The listing builds one solid part. Answer for the finished solid, in the listing's coordinates (mm). A direction names the side the tool comes from. Coordinates: 2 decimals unless noted, no trailing zeros. Write each loop counter-clockwise with the first axis right and the second up, starting at its lowest first coordinate (ties: lowest second). Pieces come first, ordered by that corner, then holes. Notation, with made-up numbers: M -35,27 L -1,27 A26 ccw -1,42 Z; hole C -30.5,17 d3. An arc over 180 degrees is marked long. Write item = value, one per line. Start each with the question number.
Autodesk Inventor part; units mm, degrees
ref_plane "YZ Plane" through (0, 0, 0) normal (1, 0, 0) x (0, 1, 0)
ref_plane "XZ Plane" through (0, 0, 0) normal (0, 1, 0) x (-1, 0, 0)
ref_plane "XY Plane" through (0, 0, 0) normal (0, 0, 1) x (1, 0, 0)
sketch "Sketch14" plane through (0, 0, 0) normal (0, 1, 0) x (-1, 0, 0)
  line L0 (0, 0) -> (0, -45.5)
  line L1 (0, -45.5) -> (-25, -45.5)
  line L2 (-25, -45.5) -> (-25, -40.4)
  line L3 (-25, -40.4) -> (-37, -40.4)
  line L4 (-33, 0) -> (0, 0)
  line L5 (0, 4) -> (4, 4)
  line L6 (4, 4) -> (4, -45.5)
  line L7 (4, -45.5) -> (4, -49.5)
  line L8 (4, -49.5) -> (-25, -49.5)
  line L9 (-37, -40.4) -> (-37, -44.4)
  line L10 (-33, 0) -> (-37, 0)
  line L11 (-37, 0) -> (-37, 4)
  line L12 (-37, 4) -> (0, 4)
  line L13 (-37, -44.4) -> (-29, -44.4)
  line L14 (-29, -44.4) -> (-25, -49.5)
  dimension "d59" = 45.5
  dimension "d60" = 25
  dimension "d61" = 5.1
  dimension "d62" = 12
  dimension "d64" = 4
  dimension "d65" = 4
  dimension "d66" = 4
  dimension "d67" = 4
  dimension "d68" = 8
extrude "Extrusion10" add sketch "Sketch14" along normal blind 35
sketch "Sketch17" plane through (0, 0, 0) normal (0, -1, 0) x (1, 0, 0)
  line L0 (0, -37.9754) -> (25, -40.4)
  line L1 (0, 0) -> (0, -45.5)
  line L2 (0, -37.9754) -> (0, -45.5)
  line L3 (25, -45.5) -> (0, -45.5)
  line L4 (0, -45.5) -> (25, -45.5)
  line L5 (25, -45.5) -> (25, -40.4)
  line L6 (25, -45.5) -> (25, -40.4)
  line L7 (25, -40.4) -> (0, -37.9754)
extrude "Extrusion12" add sketch "Sketch17" against normal blind 2.5
sketch "Sketch18" plane through (25, 0, -49.5) normal (0, 0, -1) x (-1, 0, 0)
  line L0 (25, 2.5) -> (25, 35)
  line L1 (25, 35) -> (-4.7, 35) construction
  line L2 (-4.7, 35) -> (-4.7, 15) construction
  line L3 (-4.7, 15) -> (25, 15) construction
  line L4 (25, 15) -> (25, 35) construction
  point P0 (25, 0)
  point P1 (-4.7, 25)
  dimension "d77" = 29.7
  dimension "d78" = 20
hole "Hole4" at (29.7, 15, -49.5) at (29.7, 25, -49.5) direction (0, 0, 1) diameter 3.5 depth 9.1 counterbore diameter 6 counterbore depth 7
sketch "Sketch19" plane through (-4, 0, 4) normal (0, 0, 1) x (1, 0, 0)
  circle A0 centre (33.7, 25) radius 1.75
  circle A1 centre (33.7, 15) radius 1.75
  point P0 (4, 0)
hole "Hole5" at (29.7, 25, 4) at (29.7, 15, 4) direction (0, 0, -1) diameter 3.5 depth 4 counterbore diameter 6 counterbore depth 2
properties part number "Swivel Arm Servo Holder"
1. The part is cut by section A-A, the plane y = 25. Write down the section's boundary in (x, z), and give its area (3 significant figures).
2. For faces 5 (the face through (19, 17, 0)), 6 (the face through (32, 15, -42.5)), 7 (the face through (25, 19, -43)), determine the directions among +Z, -Z, +X, -X, +Y, -Y from which every point of the face is accessible in a straight line to the end or side of a thin tool.
3. Straight lines are drawn through the part: L1, parallel to Y at x = 29.7, z = 2.8; L2, parallel to X at y = 25, z = -41; L3, parallel to X at y = 15, z = 1.05. For each, find the intervals that lie inside material, in ascending order. Write a range as [from, to].
4. The part is cut by section D-D, the plane x = 29.7. Count the separate pieces of the cut face and the enclosed holes in it, and give its area (4 significant figures).
5. The part is cut by section B-B, the plane x = 18. Write down the section's boundary in (y, z).
6. The part is cut by section C-C, the plane y = 5. Write down the section's boundary in (x, z), and give its area (3 significant figures).
7. Each of these flat-tipped pins is pushed along its axis until it touches: pin 1 (3 mm diameter, centred on x = 29.7, y = 25, fed in from +Z); pin 2 (6.5 mm diameter, centred on x = 34, y = 21, fed in from -Z); pin 3 (3 mm diameter, centred on x = 30.5, y = 14.5, fed in from -Z); pin 4 (5.5 mm diameter, centred on x = 29.7, y = 15, fed in from +Z). Where does it stop, or does it pass through?
8. For a pull along Y with two mould halves and no side action, classify faces 1 (the face through (32, 25, -42.5)), 2 (the face through (26.726, 24.609, -44.349)), 3 (the face through (31, 17, -40.4)), 4 (the face through (-2, 0, -27)) as pulls with the +Y half, pulls with the -Y half, needs draft (parallel to the pull), parting line crosses it, or undercut.
Solution:
q1.outline = M -4,-49.5 L 25,-49.5 L 26.7,-47.33 L 26.7,-42.5 L 27.95,-42.5 L 27.95,-40.4 L 25,-40.4 L 25,-45.5 L 0,-45.5 L 0,0 L 27.95,0 L 27.95,2 L 26.7,2 L 26.7,4 L -4,4 Z; M 31.45,-42.5 L 32.7,-42.5 L 32.7,-44.4 L 37,-44.4 L 37,-40.4 L 31.45,-40.4 Z; M 31.45,0 L 37,0 L 37,4 L 32.7,4 L 32.7,2 L 31.45,2 Z
q1.area = 479 mm^2
q2.face_5 = +X, +Y, -Y
q2.face_6 = -Z
q2.face_7 = +Y
q3.L1 = [0, 12], [18, 22], [28, 35]
q3.L2 = [-4, 0], [25, 27.95], [31.45, 37]
q3.L3 = [-4, 27.95], [31.45, 37]
q4.separate_pieces = 6
q4.enclosed_holes = 0
q4.area = 204.5 mm^2
q5.outline = M 0,-49.5 L 35,-49.5 L 35,-45.5 L 2.5,-45.5 L 2.5,-39.72 L 0,-39.72 Z; M 0,0 L 35,0 L 35,4 L 0,4 Z
q6.outline = M -4,-49.5 L 25,-49.5 L 29,-44.4 L 37,-44.4 L 37,-40.4 L 25,-40.4 L 25,-45.5 L 0,-45.5 L 0,0 L 37,0 L 37,4 L -4,4 Z
q6.area = 520 mm^2
q7.pin_1 = through
q7.pin_2 = -44.4
q7.pin_3 = -42.5
q7.pin_4 = 2
q8.face_1 = undercut
q8.face_2 = undercut
q8.face_3 = needs draft
q8.face_4 = pulls with the -Y half
